Model file for the job. Use its own axes, mm. A direction names the side the tool comes from. Give positions to 0.01 mm unless a question says otherwise; leave off trailing zeros. Order: outer loops, then holes, each group sorted by start corner. A loop starts at its lowest first (then second) coordinate and runs counter-clockwise, first axis right, second up. Notation, with made-up numbers: M 27.5,62 L 42.5,62 A5 ccw 42.5,68 Z; hole C 24.25,17 d11. An arc over 180 degrees is marked long. Return JSON: item names as keys, results as strings. Group by question number.
1. Slice it at B-B on y = 22. List the corners of the cut face in (x, z).
2. Wall check: probe 1 along Y at (x, z) = (31, 1.9); probe 2 along X at (y, z) = (21, 0.7); probe 3 along Y at (x, z) = (16.5, 1.5). Give the ranges that are in metal, low to high. Write a range as [from, to].
3. Two-plate mould, pull along X, no slides. Class faces 1 (the face through (39.972, 34, 2)), 2 (the face through (22, 15, 3)), 3 (the face through (30, 32.753, 1)): released by +X, released by -X, zero draft, split by the parting line, or undercut.
4. 3-axis set-ups, long thin cutter, end or side, ignore diameter. For faces 4 (the face through (29.363, 24.338, 1.479)), 5 (the face through (3.5, -1, 1)), 6 (the face through (36.972, 34, 1)): which of +Z, -Z, +X, -X, +Y, -Y reach the whole face in a straight line?
5. Pin check, flat tips, straight feed: pin 1 (1.5 mm diameter, centred on y = 34.5, z = 1, fed in from +X); pin 2 (0.9 mm diameter, centred on x = 2, z = 1, fed in from -Y); pin 3 (0.9 mm diameter, centred on y = 34.5, z = 2, fed in from -X). Stop position of each tip, or through.
6. Slice it at D-D on x = 12. List the corners of the cut face in (y, z).
7. Slice it at A-A on x = 32. List the corners of the cut face in (y, z).
8. Slice it at C-C on z = 0.7. Give the number of separate pieces and of enclosed holes in the cut face, then the cut area to 3 significant figures.
Autodesk Inventor part; units mm, degrees
ref_plane "YZ Plane" through (0, 0, 0) normal (1, 0, 0) x (0, 1, 0)
ref_plane "XZ Plane" through (0, 0, 0) normal (0, 1, 0) x (-1, 0, 0)
ref_plane "XY Plane" through (0, 0, 0) normal (0, 0, 1) x (1, 0, 0)
sketch "Esboço1" plane through (0, 0, 0) normal (0, 0, 1) x (1, 0, 0)
  line L0 (0, 0) -> (16.4719, 32.7528)
  line L1 (16.4719, 32.7528) -> (43.4719, 32.7528)
  line L2 (0, 0) -> (27, 0)
  line L3 (27, 0) -> (43.4719, 32.7528)
  line L4 (16.9941, 27.1139) -> (6.9771, 7.1962)
  line L5 (35.4733, 29.7528) -> (20.1912, 29.7528)
  line L6 (23.2808, 3) -> (7.9986, 3)
  line L7 (36.4948, 25.5566) -> (26.4779, 5.6389)
  arc A0 (7.8433, 3.4459) -> (7.9986, 3) centre (7.9986, 3.25) ccw
  arc A1 (6.9771, 7.1962) -> (7.3558, 6.888) centre (7.2005, 7.0839) ccw
  arc A2 (36.4948, 25.5566) -> (36.1161, 25.8648) centre (36.2715, 25.6689) ccw
  arc A3 (35.6286, 29.3069) -> (35.4733, 29.7528) centre (35.4733, 29.5028) ccw
  arc A4 (17.4597, 27.0634) -> (16.9941, 27.1139) centre (17.2174, 27.0016) ccw
  arc A5 (20.1912, 29.7528) -> (19.9489, 29.441) centre (20.1912, 29.5028) ccw
  line L8 (17.4597, 27.0634) -> (20.002, 17.1046)
  line L9 (20.9503, 13.3898) -> (23.523, 3.3118)
  line L10 (36.1161, 25.8648) -> (23.5569, 15.9059)
  line L11 (20.5527, 13.5238) -> (7.8433, 3.4459)
  line L12 (19.9489, 29.441) -> (22.5216, 19.363)
  line L13 (23.47, 15.6482) -> (26.0123, 5.6894)
  line L14 (35.6286, 29.3069) -> (22.9192, 19.229)
  line L15 (19.9151, 16.8469) -> (7.3558, 6.888)
  arc A6 (20.9503, 13.3898) -> (20.5527, 13.5238) centre (20.7081, 13.3279) ccw
  arc A7 (19.9151, 16.8469) -> (20.002, 17.1046) centre (19.7597, 17.0428) ccw
  arc A8 (22.5216, 19.363) -> (22.9192, 19.229) centre (22.7639, 19.4249) ccw
  arc A9 (23.5569, 15.9059) -> (23.47, 15.6482) centre (23.7122, 15.71) ccw
  arc A10 (23.2808, 3) -> (23.523, 3.3118) centre (23.2808, 3.25) ccw
  arc A11 (26.0123, 5.6894) -> (26.4779, 5.6389) centre (26.2545, 5.7512) ccw
extrude "Extrusão1" add sketch "Esboço1" along normal blind 3
sketch "Esboço2" plane through (16.4719, 32.7528, 0) normal (0, 1, 0) x (1, 0, 0)
  line L0 (27, 0) -> (0, 0)
  line L1 (27, -3) -> (0, -3)
  line L2 (23.5, 0) -> (20.5, 0)
  line L3 (20.5, 0) -> (20.5, -3)
  line L4 (20.5, -3) -> (23.5, -3)
  line L5 (23.5, -3) -> (23.5, 0)
  line L6 (3.5, 0) -> (6.5, 0)
  line L7 (6.5, 0) -> (6.5, -3)
  line L8 (6.5, -3) -> (3.5, -3)
  line L9 (3.5, -3) -> (3.5, 0)
  point P0 (-16.4719, 0)
  point P1 (3.5, -3)
  point P2 (6.5, -3)
  point P3 (6.5, 0)
  dimension "d13" = 3
  dimension "d14" = 3
  dimension "d61" = 3
  dimension "d62" = 3
extrude "Extrusão2" add sketch "Esboço2" along normal blind 3 contours L5 L1 L3 L0 | L7 L1 L9 L0
sketch "Esboço3" plane through (0, 0, 0) normal (0, -1, 0) x (1, 0, 0)
  line L0 (3.5, 3) -> (6.5, 3)
  line L1 (6.5, 3) -> (6.5, 0)
  line L2 (6.5, 0) -> (3.5, 0)
  line L3 (3.5, 0) -> (3.5, 3)
  line L4 (23.4939, 3) -> (20.4939, 3)
  line L5 (20.4939, 3) -> (20.4939, 0)
  line L6 (20.4939, 0) -> (23.4939, 0)
  line L7 (23.4939, 0) -> (23.4939, 3)
  point P0 (0, 0)
  dimension "d65" = 3
  dimension "d66" = 3
  dimension "d67" = 3
  dimension "d68" = 3
extrude "Extrusão3" add sketch "Esboço3" along normal blind 3
properties part number "ENTRE_ASA"
Result:
{
 "1": {"outline": "M 11.06,0 L 14.42,0 L 14.42,3 L 11.06,3 Z; M 18.75,0 L 21.85,0 L 21.85,3 L 18.75,3 Z; M 26.41,0 L 31.24,0 L 31.24,3 L 26.41,3 Z; M 34.71,0 L 38.06,0 L 38.06,3 L 34.71,3 Z"},
 "2": {"probe 1": "y = [7.95, 14.63], [21.81, 25.64], [29.75, 32.75]", "probe 2": "x = [10.56, 13.92], [19.01, 22.1], [25.15, 29.98], [34.2, 37.56]", "probe 3": "y = [0, 3], [10.31, 14.14], [26.13, 32.75]"},
 "3": {"face 1": "released by +X", "face 2": "zero draft", "face 3": "undercut"},
 "4": {"face 4": "+Z, -Z", "face 5": "+Z, -Z, -X, -Y", "face 6": "+Z, -Z, +Y"},
 "5": {"pin 1": "stops at x = 39.97", "pin 2": "stops at y = 0", "pin 3": "stops at x = 19.97"},
 "6": {"outline": "M 0,0 L 3,0 L 3,3 L 0,3 Z; M 6.74,0 L 10.57,0 L 10.57,3 L 6.74,3 Z; M 17.18,0 L 23.86,0 L 23.86,3 L 17.18,3 Z"},
 "7": {"outline": "M 9.94,0 L 16.62,0 L 16.62,3 L 9.94,3 Z; M 22.6,0 L 26.43,0 L 26.43,3 L 22.6,3 Z; M 29.75,0 L 32.75,0 L 32.75,3 L 29.75,3 Z"},
 "8": {"separate pieces": "1", "enclosed holes": "4", "area": "570 mm2"}
}
